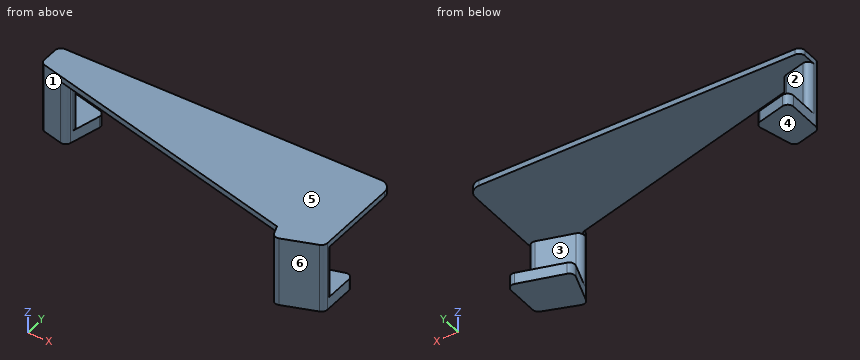
Autodesk Fusion 360 part; units mm, degrees
sketch "Sketch1" plane through (0, 0, 0) normal (0, 0, 1) x (1, 0, 0) in component "Caliper Hanging Bracket"
  line L0 (-49.4372, 12.7953) -> (0, 0)
  line L1 (8.1454, 2.4216) -> (0, 0)
  line L2 (-49.4372, 12.7953) -> (-49.4372, 17.3382)
  line L3 (-49.4372, 17.3382) -> (8.1454, 17.3382)
  line L4 (8.1454, 17.3382) -> (8.1454, 2.4216)
  line L5 (0, 0) -> (0.8806, -2.495)
  line L6 (0.8806, -2.495) -> (8.1454, 0.0691)
  line L7 (8.1454, 0.0691) -> (8.1454, 2.4216)
  line L8 (-49.4372, 12.7953) -> (-49.4372, 15.3629)
  line L9 (-49.4372, 15.3629) -> (-43.7781, 13.8982)
  line L10 (-43.7781, 13.8982) -> (-44.4009, 11.4918)
  dimension "d17" = 4.5429
  dimension "d18" = 57.5826
  dimension "d19" = 5.8456
  dimension "d20" = 51.0662
  dimension "d23" = 7.704
  dimension "d24" = 2.6458
  dimension "d25" = 8.4977
  dimension "d26" = 2.4857
extrude "Extrude1" add sketch "Sketch1" against normal blind 1 contours L0 L1 L2 L3 L4 L9 L10 makes body 1 in component "Caliper Hanging Bracket"
extrude "Extrude2" add sketch "Sketch1" against normal blind 12 contours L0 L2 L8 L9 L10 | L1 L5 L6 L7 bodies 1 in component "Caliper Hanging Bracket"
ref_plane "WorkPlane1" through (-46.6077, 13.4273, -10) normal (0, 0, -1) x (-1, 0, 0) in component "Caliper Hanging Bracket"
split "Split1" by plane through (-46.6077, 13.4273, -10) normal (0, 0, -1) bodies 1 makes body 2 at (3.0087, -0.8086, -12) makes body 3 at (-47.5509, 14.0188, -12) in component "Caliper Hanging Bracket"
move_face "OffsetFaces1" offset 5 2 faces at (-47.5509, 14.8746, -10.6667) (5.4303, 1.6144, -10.6667) on bodies 2 3 in component "Caliper Hanging Bracket"
combine "Combine1" operation add target body 1 tool bodies 2 3 in component "Caliper Hanging Bracket"
fillet "Fillet1" radius 1 13 edges at (8.1454, 7.6379, -11) (-49.4372, 17.3382, -0.5) (-49.4372, 20.5276, -11) (-49.4372, 15.3629, -5.5) (-49.4372, 12.7953, -6) (-44.4009, 11.4918, -6.5) (-43.7781, 13.8982, -5.5) (8.1454, 0.0691, -6) (8.1454, 2.4216, -5.5) (0.8806, -2.495, -6) (-1.6662, 4.7209, -11) (0, 0, -5.5) (-42.5253, 18.7387, -11) on bodies 1 in component "Caliper Hanging Bracket"
fillet "Fillet2" radius 2 1 edges at (8.1454, 17.3382, -0.5) on bodies 1 in component "Caliper Hanging Bracket"
component "Caliper Hanging Bracket" placed x (1, 0, 0) y (0, 1, 0) z (0, 0, 1) at (0, 0, 0)
Verification items for the finished model (mm, model axes). Face numbers are marked on the shaded views. A direction names the side the tool comes from. Coordinates: 2 decimals unless noted, no trailing zeros. Order: outer loops, then holes, each group sorted by start corner. A loop starts at its lowest first (then second) coordinate and runs counter-clockwise, first axis right, second up. Notation, with made-up numbers: (45.25, -7.5) -> (87.25, -7.5) arc R21 cw to (87.25, 15.5) -> close; hole circle Ø3 at (75.25, 0.25). An arc over 180 degrees is marked (long way). Put each result on its own line as item: value. Start each with the question number.
1. Access from +Z, -Z, +X, -X, +Y, -Y to the whole of each face (thin tool, end or side, straight path). Record for the marked faces 1 and 2.
2. Go/stop test with flat-tipped pins: pin 1 Ø9 at (x, y) = (5, 3.5) entering from +Z; pin 2 Ø0.5 at (x, z) = (-9.5, -0.5) entering from +Y; pin 3 Ø2 at (x, z) = (-35, -3.5) entering from +Y; pin 4 Ø4 at (x, y) = (2, 8.5) entering from -Z. Record where each tip stops, or that it passes through.
3. Cross-section at C-C, the plane y = 10. Record the boundary of the cut face in (x, z).
4. Material ranges on L1, parallel to Z at x = -32, y = 12.25; L2, parallel to X at y = 14, z = -7.25; L3, parallel to Y at x = -16.5, z = -0.5, recorded low to high. Write a range as [from, to].
5. Cross-section at A-A, the plane z = -8.5. Record the boundary of the cut face in (x, y).
6. Cross-section at B-B, the plane x = -9.5. Record the boundary of the cut face in (y, z).
7. Mould release check, pull along Z, two halves, no side actions. Record for the marked faces 3, 4, 5 and 6: released by +Z, released by -Z, zero draft, split by the parting line, or undercut.
Computed:
1. face 1: +Z, -Z, -X, -Y
1. face 2: +X, +Y
2. pin 1: z = 0
2. pin 2: y = 17.34
2. pin 3: through
2. pin 4: z = -1
3. outline: (-38.64, -1) -> (8.15, -1) -> (8.15, 0) -> (-38.64, 0) -> close
4. L1: [-1, 0]
4. L2: [-49.44, -44.42]
4. L3: [4.27, 17.34]
5. outline: (-49.44, 13.57) arc R1 ccw to (-48.69, 12.6) -> (-45.37, 11.74) arc R1 ccw to (-44.15, 12.46) -> (-44.03, 12.93) arc R1 ccw to (-44.75, 14.15) -> (-48.19, 15.04) arc R1 ccw to (-49.44, 14.07) -> close; (0.35, -0.99) -> (0.55, -1.55) arc R1 ccw to (1.82, -2.16) -> (7.48, -0.17) arc R1 ccw to (8.15, 0.78) -> (8.15, 1.08) arc R1 ccw to (6.86, 2.04) -> (1.01, 0.3) arc R1 ccw to start
6. outline: (2.46, -1) -> (17.34, -1) -> (17.34, 0) -> (2.46, 0) -> close
7. face 3: undercut
7. face 4: released by -Z
7. face 5: released by +Z
7. face 6: zero draft
